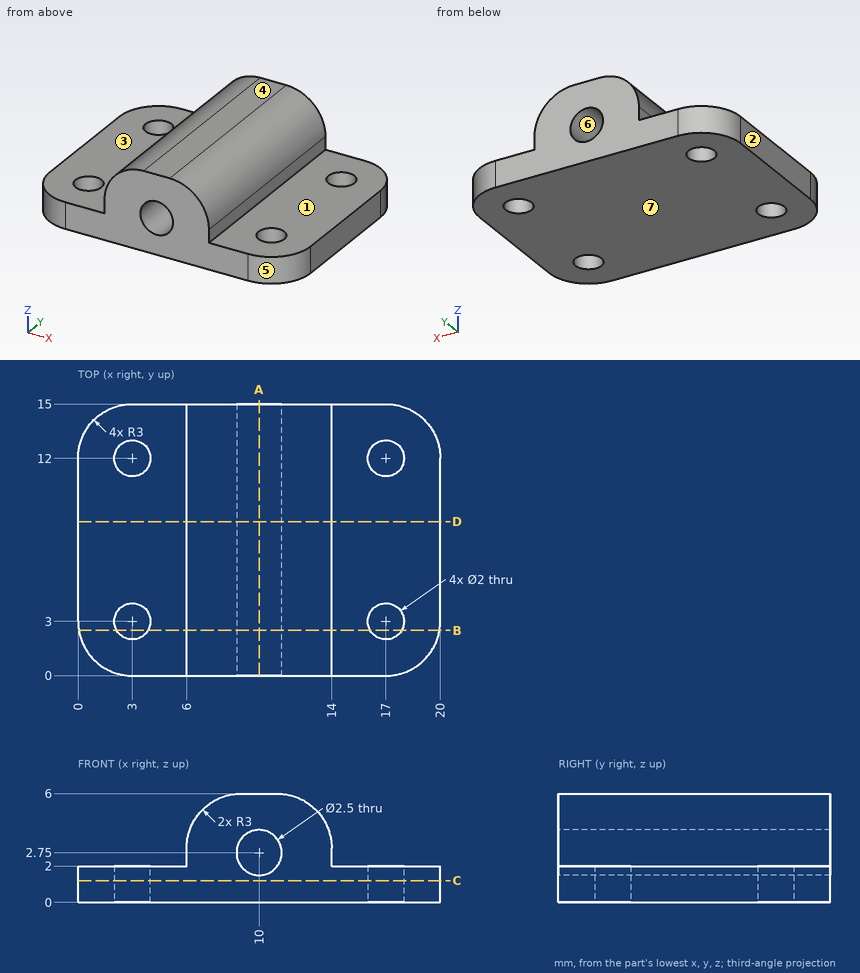
Could you check a few things on this drawing? It's one solid part, dimensions in mm from its lowest x, y, z. A direction names the side the tool comes from. Give positions to 0.01 mm unless a question says otherwise; leave off trailing zeros. Write each loop counter-clockwise with the first axis right and the second up, starting at its lowest first coordinate (ties: lowest second). Pieces come first, ordered by that corner, then holes. Notation, with made-up numbers: M 88.5,54 L 92.5,54 A23 ccw 92.5,67 Z; hole C 73,75.5 d6. An arc over 180 degrees is marked long. Put each result on its own line as item: value. Start each with the question number.
Item 1: I need wall thicknesses on L1, parallel to X at y = 12, z = 0.95; L2, parallel to Y at x = 17, z = 1; L3, parallel to X at y = 3.75, z = 1.3. Which ranges of each line are inside material? Lowest first, please. Write a range as from..to.
Item 2: Will these pins go through, and if not, where does the flat tip stop? pin 1 (1 mm diameter, centred on y = 4, z = 4.5, fed in from -X); pin 2 (3 mm diameter, centred on x = 17, y = 12, fed in from +Z); pin 3 (6.5 mm diameter, centred on x = 16, y = 10.5, fed in from +Z); pin 4 (1.8 mm diameter, centred on x = 3, y = 3, fed in from +Z).
Item 3: If we section it at D-D, the plane y = 8.5: Write out the boundary of the cut face in (x, z).
Item 4: Thinking about a two-plate mould opening in Z: for the marked faces 4, 5, 6 and 7, which applies, +Z half, -Z half, draft (parallel to the pull), parting line (faces both ways), or undercut?
Item 5: If we section it at A-A, the plane x = 10: Write out the boundary of the cut face in (y, z), then the cut area to 3 significant figures.
Item 6: If we section it at B-B, the plane y = 2.5: Write out the boundary of the cut face in (x, z), then the cut area to 3 significant figures.
Item 7: On a 3-axis mill with a long thin cutter (end or side, diameter ignored), from which of +Z, -Z, +X, -X, +Y, -Y can I reach the whole of each face in a straight line? I mean the marked faces 1, 2 and 3. Say none if no direction works.
Item 8: If we section it at C-C, the plane z = 1.2: Write out the boundary of the cut face in (x, y).
Values:
1. L1: 0..2, 4..16, 18..20
1. L2: 0..2, 4..11, 13..15
1. L3: 0..2.34, 3.66..16.34, 17.66..20
2. pin 1: x = 6.17
2. pin 2: z = 2
2. pin 3: z = 5.44
2. pin 4: through
3. outline: M 0,0 L 20,0 L 20,2 L 14,2 L 14,3 A3 ccw 11,6 L 9,6 A3 ccw 6,3 L 6,2 L 0,2 Z; hole C 10,2.75 d2.5
4. face 4: +Z half
4. face 5: draft
4. face 6: undercut
4. face 7: -Z half
5. outline: M 0,0 L 15,0 L 15,1.5 L 0,1.5 Z; M 0,4 L 15,4 L 15,6 L 0,6 Z
5. area: 52.5 mm²
6. outline: M 0.04,0 L 2.13,0 L 2.13,2 L 0.04,2 Z; M 3.87,0 L 16.13,0 L 16.13,2 L 14,2 L 14,3 A3 ccw 11,6 L 9,6 A3 ccw 6,3 L 6,2 L 3.87,2 Z; M 17.87,0 L 19.96,0 L 19.96,2 L 17.87,2 Z; hole C 10,2.75 d2.5
6. area: 56.1 mm²
7. face 1: +Z, +X, +Y, -Y
7. face 2: +Z, -Z, -X, +Y, -Y
7. face 3: +Z, -X, +Y, -Y
8. outline: M 0,3 A3 ccw 3,0 L 17,0 A3 ccw 20,3 L 20,12 A3 ccw 17,15 L 3,15 A3 ccw 0,12 Z; hole C 3,3 d2; hole C 3,12 d2; hole C 17,3 d2; hole C 17,12 d2
